CAD build for the part. Positions are in the model's coordinates, mm. Face numbers are marked on the shaded views. A direction names the side the tool comes from. Coordinates: 2 decimals unless noted, no trailing zeros. Order: outer loops, then holes, each group sorted by start corner. A loop starts at its lowest first (then second) coordinate and runs counter-clockwise, first axis right, second up. Notation, with made-up numbers: (80, 82) - (101, 82) arc R9 cw to (101, 99) - close; hole circle Ø11 at (42.5, 50.5). An arc over 180 degrees is marked (long way). Return JSON: item names as keys, results as strings.
from build123d import *

# Parameters (mm, degrees)
SKETCH_1_W               = 185
SKETCH_1_H               = 40
EXTRUDE_1_DEPTH          = 4
CUT_EXTRUDE_1_DEPTH      = 95.721961551
CUT_EXTRUDE_1_DEPTH_BACK = 95.721961551
SKETCH_2_R               = 2
SKETCH_3_W               = 10
SKETCH_3_H               = 40
EXTRUDE_2_DEPTH          = 50
EXTRUDE_3_DEPTH          = 20
CUT_EXTRUDE_2_DEPTH      = 108.033873143
CUT_EXTRUDE_2_DEPTH_BACK = 108.033873143
SKETCH_5_W               = 50
SKETCH_5_H               = 15
FILLET_1_R               = 10
FILLET_2_R               = 4
FILLET_3_R               = 2


with BuildPart() as part:
    # 草图1 → 凸台-拉伸1 (new body)
    with BuildSketch(Plane(origin=(0, 0, 0), x_dir=(1, 0, 0), z_dir=(0, 1, 0))):
        Rectangle(SKETCH_1_W, SKETCH_1_H)
    extrude(amount=-EXTRUDE_1_DEPTH)

    # 草图2 → 切除-拉伸1 (cut, two sides: drawn at the far end of the back side and taken through both)
    with BuildSketch(Plane(origin=(0, 0, 0), x_dir=(1, 0, 0), z_dir=(0, 1, 0)).offset(-CUT_EXTRUDE_1_DEPTH_BACK)):
        with Locations(Location((-75, 11.85, 0), (0, 0, 270))):
            Circle(SKETCH_2_R)
        with Locations(Location((-65, -11.85, 0), (0, 0, 270))):
            Circle(SKETCH_2_R)
        with Locations(Location((-85, -11.85, 0), (0, 0, 270))):
            Circle(SKETCH_2_R)
        with Locations(Location((65, -11.85, 0), (0, 0, 270))):
            Circle(SKETCH_2_R)
        with Locations(Location((85, -11.85, 0), (0, 0, 270))):
            Circle(SKETCH_2_R)
        with Locations(Location((75, 11.85, 0), (0, 0, 270))):
            Circle(SKETCH_2_R)
    extrude(amount=CUT_EXTRUDE_1_DEPTH + CUT_EXTRUDE_1_DEPTH_BACK, mode=Mode.SUBTRACT)

    # 草图3 → 凸台-拉伸2 (add)
    with BuildSketch(Plane(origin=(0, 0, 0), x_dir=(1, 0, 0), z_dir=(0, 1, 0))):
        Rectangle(SKETCH_3_W, SKETCH_3_H)
    extrude(amount=EXTRUDE_2_DEPTH)

    # 草图4 → 凸台-拉伸3 (add, symmetric)
    with BuildSketch(Plane.XY):
        Polygon((-5, 0), (-5, 15), (-55, 0), align=None)
        Polygon((5, 15), (55, 0), (5, 0), align=None)
    extrude(amount=EXTRUDE_3_DEPTH, both=True)

    # 草图5 → 切除-拉伸2 (cut, two sides: drawn at the far end of the back side and taken through both)
    with BuildSketch(Plane(origin=(0, 0, 0), x_dir=(1, 0, 0), z_dir=(0, 1, 0)).offset(-CUT_EXTRUDE_2_DEPTH_BACK)):
        with Locations((-30, 0)):
            Rectangle(SKETCH_5_W, SKETCH_5_H)
        Polygon((-81.842684811, 0.77750414), (-75, -13.85), (-68.157315189, 0.77750414), align=None)
        Polygon((75, -13.85), (68.157315189, 0.77750414), (81.842684811, 0.77750414), align=None)
        with Locations((30, 0)):
            Rectangle(SKETCH_5_W, SKETCH_5_H)
    extrude(amount=CUT_EXTRUDE_2_DEPTH + CUT_EXTRUDE_2_DEPTH_BACK, mode=Mode.SUBTRACT)

    # 圆角1
    fillet_1_edges = [part.edges().sort_by_distance(p)[0] for p in [
        (0, 50, -20),
        (0, 50, 20),
    ]]
    fillet(fillet_1_edges, radius=FILLET_1_R)

    # 圆角2
    fillet_2_edges = [part.edges().sort_by_distance(p)[0] for p in [
        (92.5, -2, 20),
        (-92.5, -2, 20),
        (-92.5, -2, -20),
        (92.5, -2, -20),
    ]]
    fillet(fillet_2_edges, radius=FILLET_2_R)

    # 圆角3
    fillet_3_edges = [part.edges().sort_by_distance(p)[0] for p in [
        (-81.842684811, -2, -0.77750414),
        (-68.157315189, -2, -0.77750414),
        (-75, -2, 13.85),
        (81.842684811, -2, -0.77750414),
        (75, -2, 13.85),
        (68.157315189, -2, -0.77750414),
    ]]
    fillet(fillet_3_edges, radius=FILLET_3_R)


solid = part.part
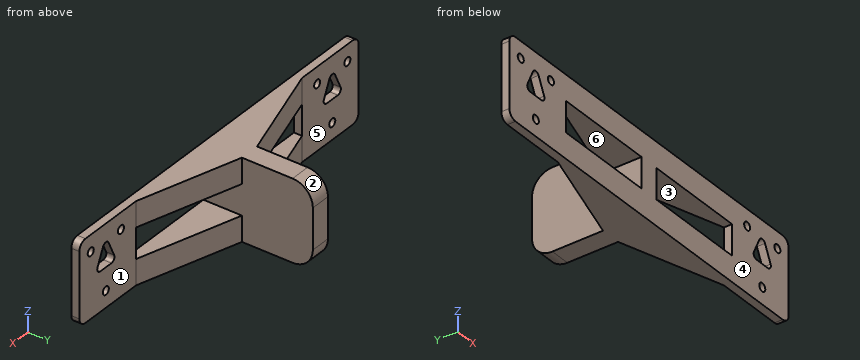
Item 1: Band-saw the part on A-A, the plane x = -52. List the corners of the cut face in (y, z).
Findings below:
{"outline": "(-4, -20) - (0.9, -20) - (0.9, -7.5) - (-4, -7.5) - close; (-4, 7.5) - (0.9, 7.5) - (0.9, 20) - (-4, 20) - close"}
Item 2: Band-saw the part on B-B, the plane z = -4. List the corners of the cut face in (x, y).
Findings below:
{"outline": "(-92.5, -4) - (-55, -4) - (-55, 0) - (-92.5, 0) - close; (-5, -4) - (5, -4) - (5, 50) - (-5, 50) - close; (55, -4) - (92.5, -4) - (92.5, 0) - (55, 0) - close"}
Item 3: Band-saw the part on D-D, the plane y = 6. List the corners of the cut face in (x, z).
Findings below:
{"outline": "(-35, -20) - (35, -20) - (35, -7.5) - (5, -7.5) - (5, 7.5) - (35, 7.5) - (35, 20) - (-35, 20) - (-35, 7.5) - (-5, 7.5) - (-5, -7.5) - (-35, -7.5) - close"}
Item 4: Mould opens along Z. For the marked faces 1, 2 and 3 say: released by +Z, released by -Z, zero draft, split by the parting line, or undercut.
Findings below:
{"face 1": "zero draft", "face 2": "released by +Z", "face 3": "undercut"}
Item 5: Drop flat-ended pins along their axis: P1, Ø10, axis at x = 61, z = 0.5, coming from the +Y side; P2, Ø12, axis at y = 35, z = 0.5, coming from the -X side; P3, Ø10, axis at x = -58, z = -7.5, coming from the +Y side. Give the stop position or say it passes through.
Findings below:
{"P1": "stops at y = 0", "P2": "stops at x = -5", "P3": "stops at y = 0.6"}
Item 6: Wall check: L1, parallel to X at y = -2.8, z = 11.85; L2, parallel to Z at x = 75, y = -2.5; L3, parallel to X at y = -1.7, z = -11.85. Give the ranges that are in metal, low to high. Write a range as [from, to].
Findings below:
{"L1": "x = [-92.5, -87], [-83, -67], [-63, 63], [67, 83], [87, 92.5]", "L2": "z = [-20, -13.85], [-9.85, -0.78], [11.13, 20]", "L3": "x = [-92.5, -77], [-73, 73], [77, 92.5]"}
Item 7: Band-saw the part on C-C, the plane x = -26.5. List the corners of the cut face in (y, z).
Findings below:
{"outline": "(-4, -20) - (8.55, -20) - (8.55, -7.5) - (-4, -7.5) - close; (-4, 7.5) - (8.55, 7.5) - (8.55, 20) - (-4, 20) - close"}
Item 8: Which spindle directions (+Z, -Z, +X, -X, +Y, -Y) get a long thin tool onto all of the face, cutting with end or side? Do the marked faces 4, 5 and 6. Say none if no direction does.
Findings below:
{"face 4": "+Z, -Z, +X, -X, -Y", "face 5": "+Z, -Z, -X, +Y", "face 6": "+Y, -Y"}
